```python
from build123d import *

# Parameters (mm, degrees)
F0_W     = 25.4
F0_H     = 25.4
F1_DEPTH = 25.4
F2_R     = 1.27
F3_DEPTH = 12.7
F5_DEPTH = 22.86
F6_R     = 2.54


with BuildPart() as f1:
    # F0 (on Top) → F1 (new body)
    with BuildSketch(Plane.XY):
        with Locations((12.7, 12.7)):
            Rectangle(F0_W, F0_H)
    extrude(amount=F1_DEPTH)

    # F2 (on face) → F3 (cut)
    with BuildSketch(Plane.XY.offset(25.4)):
        with Locations((22.86, 22.86)):
            Circle(F2_R)
    extrude(amount=-F3_DEPTH, mode=Mode.SUBTRACT)

    # F4 (on face) → F5 (cut)
    with BuildSketch(Plane.XY.offset(25.4)):
        Polygon((24.13, 1.27), (24.13, 20.32), (20.32, 20.32), (20.32, 24.13), (1.27, 24.13), (1.27, 1.27), align=None)
    extrude(amount=-F5_DEPTH, mode=Mode.SUBTRACT)

    # F6
    f6_edges = [f1.edges().sort_by_distance(p)[0] for p in [
        (20.32, 20.32, 13.97),
    ]]
    fillet(f6_edges, radius=F6_R)


solid = f1.part
```
Check sheet for the modelled part. Datum: model origin and axes. Units: mm. A direction names the side the tool comes from. Coordinates: 2 decimals unless noted, no trailing zeros. Loops run counter-clockwise (first coordinate to the right, second up) from the corner with the lowest first, then second, coordinate; pieces in that order, holes last.
1) Gauge pin test, flat ends, axial feed: pin 1 (5.5 mm diameter, centred on y = 7.5, z = 14, fed in from -X); pin 2 (5 mm diameter, centred on x = 8, y = 21, fed in from +Z). Record the tip position at first contact, or that the pin passes through.
2) Release check for a two-part mould opening along X. For faces 3 (the face through (0, 13, 13)), 4 (the face through (13, 13, 0)), 5 (the face through (21.084, 21.044, 13.81)) record: released by +X, released by -X, zero draft, split by the parting line, or undercut.
3) Sectioned sample at C-C (z = 15.5). Record the boundary of the cut face in (x, y).
4) Material ranges on probe 1 along Y at (x, z) = (22.86, 16.5); probe 2 along Y at (x, z) = (15.25, 14), recorded low to high.
5) Sectioned sample at A-A (z = 10.25). Record the boundary of the cut face in (x, y).
6) Access from +Z, -Z, +X, -X, +Y, -Y to the whole of each face (thin tool, end or side, straight path). Record for faces 1 (the face through (23, 23, 12.7)), 2 (the face through (13, 0, 13)).
7) Sectioned sample at B-B (y = 5.5). Record the boundary of the cut face in (x, z), and give its area (3 significant figures).
Check sheet entries:
1. pin 1: stops at x = 0
1. pin 2: stops at z = 2.54
2. face 3: released by -X
2. face 4: zero draft
2. face 5: undercut
3. outline: (0, 0) - (25.4, 0) - (25.4, 25.4) - (0, 25.4) - close; hole (1.27, 1.27) - (24.13, 1.27) - (24.13, 20.32) - (22.86, 20.32) arc R2.54 cw to (20.32, 22.86) - (20.32, 24.13) - (1.27, 24.13) - close; hole circle Ø2.54 at (22.86, 22.86)
4. probe 1: y = 0 to 1.27, 20.32 to 21.59, 24.13 to 25.4
4. probe 2: y = 0 to 1.27, 24.13 to 25.4
5. outline: (0, 0) - (25.4, 0) - (25.4, 25.4) - (0, 25.4) - close; hole (1.27, 1.27) - (24.13, 1.27) - (24.13, 20.32) - (22.86, 20.32) arc R2.54 cw to (20.32, 22.86) - (20.32, 24.13) - (1.27, 24.13) - close
6. face 1: +Z
6. face 2: +Z, -Z, +X, -X, -Y
7. outline: (0, 0) - (25.4, 0) - (25.4, 25.4) - (24.13, 25.4) - (24.13, 2.54) - (1.27, 2.54) - (1.27, 25.4) - (0, 25.4) - close
7. area: 123 mm2
